Solid Edge part; units mm, degrees
sketch "Sketch1" plane through (0, 0, 0) normal (0, 0, 1) x (1, 0, 0)
  line L0 (0, 45.5) -> (0, 6.5)
  line L1 (13, 6.5) -> (13, 45.5)
  arc A0 (13, 6.5) -> (0, 6.5) centre (6.5, 6.5) cw
  arc A1 (0, 45.5) -> (13, 45.5) centre (6.5, 45.5) cw
extrude "Protrusion1" add sketch "Sketch1" along normal blind 6.5
sketch "Sketch2" plane through (6.5, 0, 0) normal (1, 0, 0) x (0, 1, 0)
  line L0 (3.5, 5.5) -> (3.5, 6.5)
  line L1 (3.5, 6.5) -> (6.5, 6.5)
  line L2 (6.5, 1) -> (6.5, 6.5)
  line L3 (3.5, 1) -> (6.5, 1)
  line L4 (3.5, 1) -> (2.6811, 3.25)
  line L5 (3.5, 5.5) -> (2.6811, 3.25)
revolve "RevolvedCutout1" cut sketch "Sketch2" angle 360 about axis through (6.5, 6.5, 1) along (0, 0, 1)
chamfer "Chaflán_38" distance 0.75 angle 45 1 edges at (6.5, 3.5, 6.5)
pattern_linear "Pattern1" count 4 spacing 13 along (0, 1, 0) of "RevolvedCutout1", "Chaflán_38"
chamfer "Chaflán_39" distance 1.5 angle 45 8 edges at (13, 26, 6.5) (6.5, 0, 6.5) (0, 26, 6.5) (6.5, 52, 6.5) (13, 26, 0) (6.5, 0, 0) (0, 26, 0) (6.5, 52, 0)
For this review, take the finished solid that the model builds, in its own axes (mm). A direction names the side the tool comes from. Coordinates: 2 decimals unless noted, no trailing zeros. Order: outer loops, then holes, each group sorted by start corner. A loop starts at its lowest first (then second) coordinate and runs counter-clockwise, first axis right, second up. Notation, with made-up numbers: (-27, 10.5) - (12, 10.5) arc R22 ccw to (12, 44.5) - close; hole circle Ø8 at (6, 40.5). An arc over 180 degrees is marked (long way). Answer as a JSON object with one key per item and string values. Group by question number.
1. The part is to be moulded in two halves that separate along X. For faces 4 (the cylindrical face through (6.4, 52, 3.2)), 5 (the conical face through (8.357, 8.921, 5.359)), 6 (the flat face through (0, 26, 3)), 7 (the flat face through (6, 26, 0)), say which applies: pulls with the +X half, pulls with the -X half, needs draft (parallel to the pull), parting line crosses it, or undercut.
2. We need section C-C on z = 0.5. State the section outline as (x, y) points, then the cut area to 3 significant figures.
3. For faces 1 (the conical face through (6.4, 1.2, 0.3)), 2 (the conical face through (7.669, 42.681, 5.359)), 3 (the flat face through (7, 46, 1)), list the 3-axis set-ups (+Z, -Z, +X, -X, +Y, -Y) from which the entire face can be reached by the end or side of a thin tool; tool diameter is ignored.
4. We need section A-A on y = 39. State the section outline as (x, z) points.
5. For probe 1 along Y at (x, z) = (8.5, 4.5); probe 2 along Y at (x, z) = (5.25, 5.5); probe 3 along X at (y, z) = (45, 2.25), list the stretches that pass through material, from the lowest coordinate up.
6. We need section B-B on z = 2.5. State the section outline as (x, y) points.
7. Clearance check with flat-ended pins moving along their axes: P1, Ø6.5, axis at x = 5.5, y = 31, coming from the +Z side; P2, Ø1.5, axis at x = 2.5, z = 2, coming from the -Y side; P3, Ø3, axis at x = 4, z = 1, coming from the +Y side; P4, Ø1.8, axis at x = 7, y = 18.5, coming from the +Z side. State where each tip first meets the part, or that it passes through.
8. We need section D-D on y = 32.5. State the section outline as (x, z) points, then the cut area to 3 significant figures.
Final values:
{
 "1": {"face 4": "parting line crosses it", "face 5": "undercut", "face 6": "pulls with the -X half", "face 7": "needs draft"},
 "2": {"outline": "(1, 6.5) arc R5.5 ccw to (12, 6.5) - (12, 45.5) arc R5.5 ccw to (1, 45.5) - close", "area": "524 mm²"},
 "3": {"face 1": "-Z, -Y", "face 2": "none", "face 3": "+Z"},
 "4": {"outline": "(0, 1.5) - (1.5, 0) - (11.5, 0) - (13, 1.5) - (13, 5) - (11.5, 6.5) - (1.5, 6.5) - (0, 5) - close"},
 "5": {"probe 1": "0.32 to 3.8, 9.2 to 16.8, 22.2 to 29.8, 35.2 to 42.8, 48.2 to 51.68", "probe 2": "0.63 to 3.77, 9.23 to 16.77, 22.23 to 29.77, 35.23 to 42.77, 48.23 to 51.37", "probe 3": "0 to 3.08, 9.92 to 13"},
 "6": {"outline": "(0, 6.5) arc R6.5 ccw to (13, 6.5) - (13, 45.5) arc R6.5 ccw to (0, 45.5) - close; hole circle Ø7.09 at (6.5, 6.5); hole circle Ø7.09 at (6.5, 19.5); hole circle Ø7.09 at (6.5, 32.5); hole circle Ø7.09 at (6.5, 45.5)"},
 "7": {"P1": "z = 6.5", "P2": "y = 0.87", "P3": "y = 51.91", "P4": "z = 1"},
 "8": {"outline": "(0, 1.5) - (1.5, 0) - (11.5, 0) - (13, 1.5) - (13, 5) - (11.5, 6.5) - (10.25, 6.5) - (9.5, 5.75) - (9.5, 5.5) - (10.32, 3.25) - (9.5, 1) - (3.5, 1) - (2.68, 3.25) - (3.5, 5.5) - (3.5, 5.75) - (2.75, 6.5) - (1.5, 6.5) - (0, 5) - close", "area": "42.8 mm²"}
}
